Input: dimensioned drawing with shaded views. Units: mm. Origin: part minimum x, y, z. Coordinates: 2 decimals unless noted, no trailing zeros. Order: outer loops, then holes, each group sorted by start corner. A loop starts at its lowest first (then second) coordinate and runs counter-clockwise, first axis right, second up.
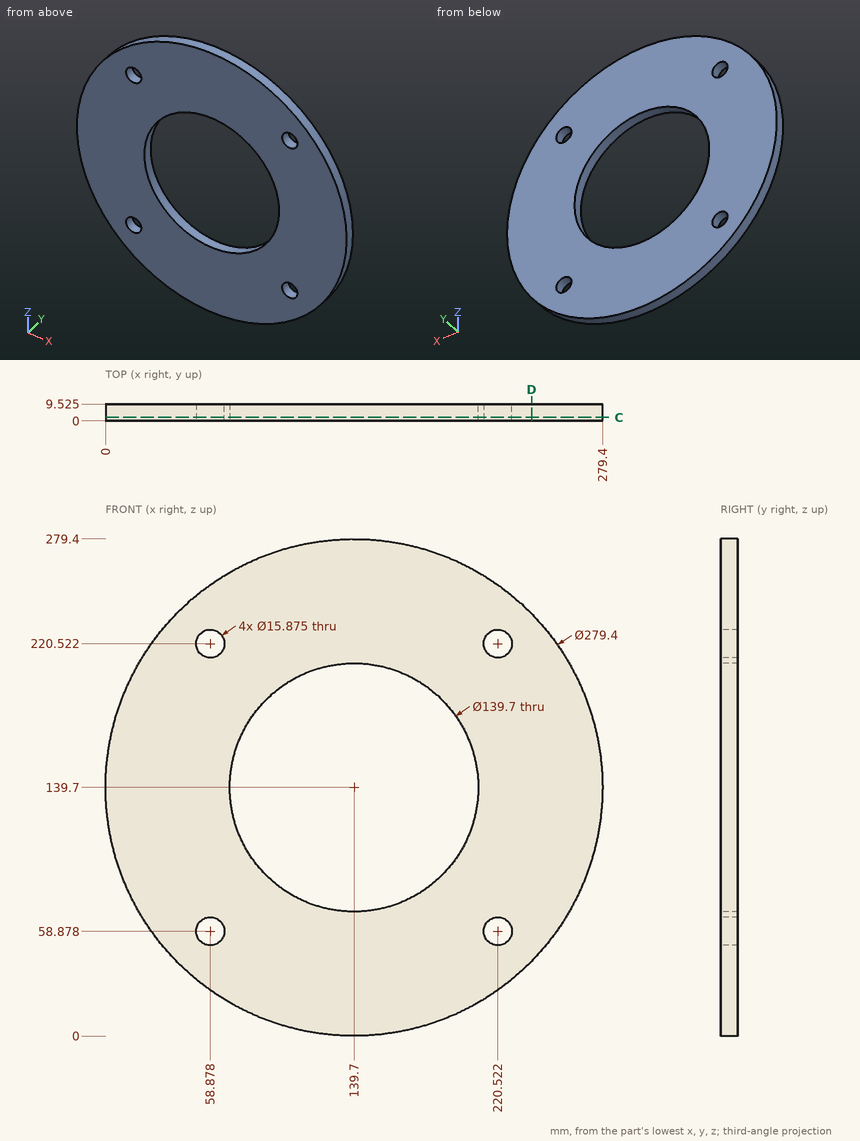
1. Section query D-D on x = 239.5. Return loops of the section in (y, z) (1 decimal), plus the area to 3 significant figures.
Findings:
outline: (0, 41.9) - (9.5, 41.9) - (9.5, 237.5) - (0, 237.5) - close
area: 1,860 mm2
2. Pin query (flat end, axial travel): P1, Ø12.5, axis at x = 220.52, z = 58.88, coming from the +Y side; P2, Ø4, axis at x = 107.5, y = 4.5, coming from the +Z side; P3, Ø1.5, axis at y = 7.5, z = 165, coming from the -X side; P4, Ø5, axis at x = 250.5, y = 7, coming from the -Z side (1 decimal). Return the tip coordinate at first contact, or that it passes through.
Findings:
P1: passes through
P2: stops at z = 276.1
P3: stops at x = 2.17
P4: stops at z = 51.5
3. Section query C-C on y = 2. Count the separate pieces of the cut face and the enclosed holes in it, plus the area to 3 significant figures.
Findings:
separate pieces: 1
enclosed holes: 5
area: 45,200 mm2
4. Ray query, line 1 (X direction, y = 4.5, z = 139.7); line 2 (X direction, y = 1.5, z = 66) (1 decimal); line 3 (Z direction, x = 224.5, y = 3). Return the intervals inside material, ascending.
Findings:
line 1: x = 0 to 69.85, 209.55 to 279.4
line 2: x = 21 to 55.4, 62.4 to 217, 224 to 258.4
line 3: z = 28.68 to 52.01, 65.75 to 213.65, 227.39 to 250.72
